Model file for the job. Use its own axes, mm. A direction names the side the tool comes from. Give positions to 0.01 mm unless a question says otherwise; leave off trailing zeros. Order: outer loops, then holes, each group sorted by start corner. A loop starts at its lowest first (then second) coordinate and runs counter-clockwise, first axis right, second up. Notation, with made-up numbers: (83, 84) - (98, 84) arc R37 ccw to (98, 123) - close; hole circle Ø1 at (-30.75, 87). An arc over 180 degrees is marked (long way). Use CSV: the item, a comma, the result in double quotes. Start each with the question number.
(1) Probe L1, parallel to X at y = 25, z = 3; L2, parallel to X at y = -6, z = 4; L3, parallel to Y at x = 0, z = 7.25. List the from-to ranges inside material, lowest first.
(2) Band-saw the part on B-B, the plane x = -20. Give the cut face in (y, z).
(3) Band-saw the part on A-A, the plane z = 7.25. Give the cut face in (x, y).
(4) Pull direction Y, two halves, no side cores. Call faces 4 (the cylindrical face through (-5.85, -26.36, 3.94)), 5 (the flat face through (6, 0, 0)), 6 (the cylindrical face through (-19.071, 26.456, 4.451)): +Y half, -Y half, draft (parallel to the pull), parting line (faces both ways), or undercut.
(5) Drop flat-ended pins along their axis: pin 1 Ø3 at (x, y) = (-20, 25) entering from -Z; pin 2 Ø5.5 at (x, y) = (-6.91, -6.91) entering from +Z; pin 3 Ø3 at (x, y) = (1.5, 1.5) entering from +Z; pin 4 Ø2 at (y, z) = (-17, 2) entering from +X. Give the stop position or say it passes through.
(6) Band-saw the part on C-C, the plane y = 25. Give the cut face in (x, z).
(7) Tool access for faces 1 (the cylindrical face through (1.43, -2.75, 2.22)), 2 (the flat face through (0.1, 27.3, 1)), 3 (the cylindrical face through (1.43, -2.75, 6.73)): list every direction of +Z, -Z, +X, -X, +Y, -Y with a clear straight run to the whole face (end or side of a thin tool).
(8) Band-saw the part on D-D, the plane y = 15. Give the cut face in (x, z), then the cut area to 3 significant figures.
from build123d import *

# Parameters (mm, degrees)
SKETCH008_R      = 27
SKETCH008_R_2    = 3.1
PAD007_DEPTH     = 8
HOLE_D           = 4.3
HOLE_CSINK_D     = 8.298
HOLE_CSINK_ANGLE = 82
SKETCH075_R      = 4
PAD048_DEPTH     = 1
PAD054_DEPTH     = 7
SKETCH089_R      = 1.7272
POCKET028_DEPTH  = 8.001


with BuildPart() as part:
    # Sketch008 → Pad007 (new body)
    with BuildSketch(Plane.XY):
        Circle(SKETCH008_R)
        Circle(SKETCH008_R_2, mode=Mode.SUBTRACT)
    extrude(amount=PAD007_DEPTH)

    # Hole (through all)
    with Locations(Plane.XY.offset(8)):
        with Locations((-6.914797, 6.914797), (6.914797, 6.914797), (6.914797, -6.914797), (-6.914797, -6.914797)):
            CounterSinkHole(HOLE_D / 2, HOLE_CSINK_D / 2, counter_sink_angle=HOLE_CSINK_ANGLE)

    # Sketch075 → Pad048 (join)
    with BuildSketch(Plane.XY.offset(4.5)):
        Circle(SKETCH075_R)
    extrude(amount=PAD048_DEPTH)

    # Sketch088 → Pad054 (join)
    with BuildSketch(Plane.XY.offset(1)):
        with BuildLine():
            Line((-27, 0), (-27, 30))
            Line((-27, 30), (27, 30))
            Line((27, 30), (27, 0))
            Line((27, 0), (26.5, 0))
            ThreePointArc((26.5, 0), (0, 26.5), (-26.5, 0))
            Line((-26.5, 0), (-27, 0))
        make_face()
    extrude(amount=PAD054_DEPTH)

    # Sketch089 → Pocket028 (cut, through all)
    with BuildSketch(Plane.XY):
        with Locations((-20, 25)):
            Circle(SKETCH089_R)
        with Locations((20, 25)):
            Circle(SKETCH089_R)
    extrude(amount=POCKET028_DEPTH, mode=Mode.SUBTRACT)


solid = part.part
Answer block:
1,L1,"x = -27 to -21.73, -18.27 to 18.27, 21.73 to 27"
1,L2,"x = -26.32 to -8.86, -4.97 to 4.97, 8.86 to 26.32"
1,L3,"y = -27 to -3.1, 3.1 to 30"
2,outline,"(-18.14, 0) - (18.14, 0) - (18.14, 1) - (23.27, 1) - (23.27, 8) - (-18.14, 8) - close; (26.73, 1) - (30, 1) - (30, 8) - (26.73, 8) - close"
3,outline,"(-27, 0) arc R27 ccw to (27, 0) - (27, 30) - (-27, 30) - close; hole circle Ø3.45 at (-20, 25); hole circle Ø6.99 at (-6.91, -6.91); hole circle Ø6.99 at (-6.91, 6.91); hole circle Ø6.2 at (0, 0); hole circle Ø6.99 at (6.91, -6.91); hole circle Ø6.99 at (6.91, 6.91); hole circle Ø3.45 at (20, 25)"
4,face 4,"parting line"
4,face 5,"draft"
4,face 6,"undercut"
5,pin 1,"passes through"
5,pin 2,"stops at z = 6.4"
5,pin 3,"stops at z = 8"
5,pin 4,"stops at x = 21.75"
6,outline,"(-27, 1) - (-21.73, 1) - (-21.73, 8) - (-27, 8) - close; (-18.27, 1) - (-10.2, 1) - (-10.2, 0) - (10.2, 0) - (10.2, 1) - (18.27, 1) - (18.27, 8) - (-18.27, 8) - close; (21.73, 1) - (27, 1) - (27, 8) - (21.73, 8) - close"
7,face 1,"-Z"
7,face 2,"-Z, +Y"
7,face 3,"+Z"
8,outline,"(-27, 1) - (-22.45, 1) - (-22.45, 0) - (22.45, 0) - (22.45, 1) - (27, 1) - (27, 8) - (-27, 8) - close"
8,area,"423 mm2"
